The model under review builds one solid part; all positions refer to its coordinate system, in mm. A direction names the side the tool comes from. Give positions to 0.01 mm unless a question says otherwise; leave off trailing zeros. Loops run counter-clockwise (first coordinate to the right, second up) from the corner with the lowest first, then second, coordinate; pieces in that order, holes last. Notation, with made-up numbers: M 63,51.25 L 89,51.25 A24 ccw 89,69.25 Z; hole C 52.5,88.25 d9. An arc over 180 degrees is marked long. Return JSON: item names as keys, results as strings.
```python
from build123d import *

# Parameters (mm, degrees)
SKETCH1_R           = 5
SKETCH1_R_2         = 17.5
SKETCH1_R_3         = 2.6
BOSS_EXTRUDE1_DEPTH = 5
FILLET1_R           = 3.5
FILLET2_R           = 2
FILLET3_R           = 0.5


with BuildPart() as part:
    # Sketch1 → Boss-Extrude1 (new body)
    # profile 1 of 4: a face of its own
    with BuildSketch(Plane.XY):
        with BuildLine():
            ThreePointArc((-9.943063938, -14.400884679), (-15.155444566, -8.75), (-17.443063938, -1.410503622))
            Line((-17.443063938, -1.410503622), (-31.895825623, -9.754809472))
            Line((-31.895825623, -9.754809472), (-24.395825623, -22.745190528))
            Line((-24.395825623, -22.745190528), (-9.943063938, -14.400884679))
        make_face()
        with Locations((-21.217622393, -12.25)):
            Circle(SKETCH1_R, mode=Mode.SUBTRACT)
    # profile 2 of 4: a face of its own
    with BuildSketch(Plane.XY):
        Circle(SKETCH1_R_2)
        Circle(SKETCH1_R_3, mode=Mode.SUBTRACT)
    # profile 3 of 4: a face of its own
    with BuildSketch(Plane.XY):
        with BuildLine():
            Line((31.895825623, -9.754809472), (17.443063938, -1.410503622))
            ThreePointArc((17.443063938, -1.410503622), (15.155444566, -8.75), (9.943063938, -14.400884679))
            Line((9.943063938, -14.400884679), (24.395825623, -22.745190528))
            Line((24.395825623, -22.745190528), (31.895825623, -9.754809472))
        make_face()
        with Locations((21.217622393, -12.25)):
            Circle(SKETCH1_R, mode=Mode.SUBTRACT)
    # profile 4 of 4: a face of its own
    with BuildSketch(Plane.XY):
        with BuildLine():
            Line((7.5, 32.5), (-7.5, 32.5))
            Line((-7.5, 32.5), (-7.5, 15.811388301))
            ThreePointArc((-7.5, 15.811388301), (0, 17.5), (7.5, 15.811388301))
            Line((7.5, 15.811388301), (7.5, 32.5))
        make_face()
        with Locations((0, 25)):
            Circle(SKETCH1_R, mode=Mode.SUBTRACT)
    extrude(amount=BOSS_EXTRUDE1_DEPTH)

    # Fillet1
    fillet1_edges = [part.edges().sort_by_distance(p)[0] for p in [
        (-24.395825623, -22.745190528, 2.5),
        (-31.895825623, -9.754809472, 2.5),
        (-7.5, 32.5, 2.5),
        (7.5, 32.5, 2.5),
        (31.895825623, -9.754809472, 2.5),
        (24.395825623, -22.745190528, 2.5),
    ]]
    fillet(fillet1_edges, radius=FILLET1_R)

    # Fillet2
    fillet2_edges = [part.edges().sort_by_distance(p)[0] for p in [
        (-17.443063938, -1.410503622, 2.5),
        (-7.5, 15.811388301, 2.5),
        (7.5, 15.811388301, 2.5),
        (17.443063938, -1.410503622, 2.5),
        (9.943063938, -14.400884679, 2.5),
        (-9.943063938, -14.400884679, 2.5),
    ]]
    fillet(fillet2_edges, radius=FILLET2_R)

    # Fillet3
    fillet3_edges = [part.edges().sort_by_distance(p)[0] for p in [
        (-2.6, 0, 5),
        (-5, 25, 5),
        (16.217622393, -12.25, 5),
        (-26.217622393, -12.25, 5),
    ]]
    fillet(fillet3_edges, radius=FILLET3_R)


solid = part.part
```
1) Tool access review of faces 1 (the face through (16.11, -17.96, 2.46)), 2 (the face through (-24.9, -8.87, 2.22)): name each direction out of +Z, -Z, +X, -X, +Y, -Y from which nothing blocks a thin tool from reaching the whole face with its end or side.
From the geometry:
{"face 1": "+Z, -Z, -Y", "face 2": "+Z, -Z"}
2) Consider section D-D on x = -14. Write out the cut boundary in (y, z), then the cut area to 3 significant figures.
From the geometry:
{"outline": "M -16.74,0 L 10.5,0 L 10.5,5 L -16.74,5 Z", "area": "136 mm²"}
3) Wall thickness on L1, parallel to X at y = -10, z = 4.65; L2, parallel to Y at x = -0.5, z = 2.2; L3, parallel to Y at x = 2, z = 4.3: over which ranges is each line inside the solid? List them lowest first. Write a range as from..to.
From the geometry:
{"L1": "-30.46..-25.71, -16.73..16.73, 25.71..30.46", "L2": "-17.49..-2.55, 2.55..20.03, 29.97..32.5", "L3": "-17.39..-1.66, 1.66..20.42, 29.58..32.5"}
4) Insertion check: pin 1 (2 mm diameter, centred on y = 13.5, z = 4, fed in from -X); pin 2 (2.5 mm diameter, centred on y = 25, z = 1.5, fed in from +X). Each pin has a flat end and moves straight along its axis. Give the tip position at first contact, or say it passes through.
From the geometry:
{"pin 1": "x = -12.25", "pin 2": "x = 7.5"}
5) Consider section B-B on z = 3. Write out the cut boundary in (x, y), then the cut area to 3 significant figures.
From the geometry:
{"outline": "M -30.15,-12.79 L -26.15,-19.71 A3.5 ccw -21.36,-21 L -11,-15.01 A2 cw -8.97,-15.02 A17.5 ccw 8.97,-15.02 A2 cw 11,-15.01 L 21.36,-21 A3.5 ccw 26.15,-19.71 L 30.15,-12.79 A3.5 ccw 28.86,-8 L 18.5,-2.02 A2 cw 17.5,-0.26 A17.5 ccw 8.53,15.28 A2 cw 7.5,17.03 L 7.5,29 A3.5 ccw 4,32.5 L -4,32.5 A3.5 ccw -7.5,29 L -7.5,17.03 A2 cw -8.53,15.28 A17.5 ccw -17.5,-0.26 A2 cw -18.5,-2.02 L -28.86,-8 A3.5 ccw Z; hole C -21.22,-12.25 d10; hole C 0,25 d10; hole C 0,0 d5.2; hole C 21.22,-12.25 d10", "area": "1,390 mm²"}
6) Consider section C-C on y = 12. Write out the cut boundary in (x, z).
From the geometry:
{"outline": "M -12.74,0 L 12.74,0 L 12.74,5 L -12.74,5 Z"}
7) Consider section A-A on x = 0. Write out the cut boundary in (y, z).
From the geometry:
{"outline": "M -17.5,0 L -2.6,0 L -2.6,4.5 A0.5 ccw -3.1,5 L -17.5,5 Z; M 2.6,0 L 20,0 L 20,4.5 A0.5 ccw 19.5,5 L 3.1,5 A0.5 ccw 2.6,4.5 Z; M 30,0 L 32.5,0 L 32.5,5 L 30.5,5 A0.5 ccw 30,4.5 Z"}
8) The part is to be moulded in two halves that separate along X. For faces 3 (the face through (6.5, 31.45, 2.54)), 4 (the face through (-1.08, 20.12, 2.22)), 5 (the face through (-28.174, -16.202, 2.465)), 6 (the face through (-16.25, -18.04, 2.46)), say which applies: released by +X, released by -X, zero draft, split by the parting line, or undercut.
From the geometry:
{"face 3": "released by +X", "face 4": "undercut", "face 5": "released by -X", "face 6": "undercut"}
